from build123d import *

# Parameters (mm, degrees)
SKETCH_2_R          = 6.5
EXTRUDE_1_DEPTH     = 2.5
SKETCH_3_R          = 2.1
CUT_EXTRUDE_1_DEPTH = 2.5
CUT_EXTRUDE_2_DEPTH = 10
SKETCH_5_R          = 2.2
CUT_EXTRUDE_3_DEPTH = 10
CUT_EXTRUDE_4_DEPTH = 10


with BuildPart() as part:
    # 草图2 → 凸台-拉伸1 (new body)
    with BuildSketch(Plane(origin=(0, 0, 0), x_dir=(1, 0, 0), z_dir=(0, 1, 0))):
        with BuildLine():
            ThreePointArc((-47.091925455, 9.778744699), (-55, -1.253e-06), (-47.091923006, -9.778745223))
            ThreePointArc((-47.091923006, -9.778745223), (-33.750000065, -19.485571473), (-32.014603203, -35.893428778))
            ThreePointArc((-32.014603203, -35.893428778), (-27.500000081, -47.631397162), (-15.077319674, -45.672174193))
            ThreePointArc((-15.077319674, -45.672174193), (-9.8e-08, -38.97114317), (15.077319542, -45.672174048))
            ThreePointArc((15.077319542, -45.672174048), (27.500000118, -47.63139714), (32.014603117, -35.893428511))
            ThreePointArc((32.014603117, -35.893428511), (33.750000078, -19.485571451), (47.091922781, -9.778745271))
            ThreePointArc((47.091922781, -9.778745271), (55, -2.05e-07), (47.091923183, 9.778745185))
            ThreePointArc((47.091923183, 9.778745185), (33.750000105, 19.485571404), (32.01460321, 35.893428798))
            ThreePointArc((32.01460321, 35.893428798), (27.499999984, 47.631397217), (15.077319539, 45.672174044))
            ThreePointArc((15.077319539, 45.672174044), (1.8e-08, 38.97114317), (-15.077319515, 45.672174018))
            ThreePointArc((-15.077319515, 45.672174018), (-27.5000001, 47.63139715), (-32.014603117, 35.893428511))
            ThreePointArc((-32.014603117, 35.893428511), (-33.750000761, 19.485570266), (-47.091925455, 9.778744699))
        make_face()
        with Locations(Location((0, 0, 0), (0, 0, 270))):
            Circle(SKETCH_2_R, mode=Mode.SUBTRACT)
    extrude(amount=EXTRUDE_1_DEPTH)

    # 草图3 → 切除-拉伸1 (cut)
    with BuildSketch(Plane(origin=(0, 2.5, 0), x_dir=(1, 0, 0), z_dir=(0, 1, 0))):
        with Locations(Location((-22.5, 38.97114317, 0), (0, 0, 270))):
            Circle(SKETCH_3_R)
        with Locations(Location((22.5, 38.97114317, 0), (0, 0, 270))):
            Circle(SKETCH_3_R)
        with Locations(Location((45, 0, 0), (0, 0, 270))):
            Circle(SKETCH_3_R)
        with Locations(Location((22.5, -38.97114317, 0), (0, 0, 270))):
            Circle(SKETCH_3_R)
        with Locations(Location((-22.5, -38.97114317, 0), (0, 0, 270))):
            Circle(SKETCH_3_R)
        with Locations(Location((-45, 0, 0), (0, 0, 270))):
            Circle(SKETCH_3_R)
    extrude(amount=-CUT_EXTRUDE_1_DEPTH, mode=Mode.SUBTRACT)

    # 草图4 → 切除-拉伸2 (cut)
    with BuildSketch(Plane(origin=(0, 2.5, 0), x_dir=(1, 0, 0), z_dir=(0, 1, 0))):
        Polygon((-21.320889551, 23.855935356), (13.529450533, 3.223344728), (3.340516889, -13.986699758), (-31.509823195, 6.64589087), align=None)
    extrude(amount=-CUT_EXTRUDE_2_DEPTH, mode=Mode.SUBTRACT)

    # 草图5 → 切除-拉伸3 (cut)
    with BuildSketch(Plane(origin=(0, 2.5, 0), x_dir=(1, 0, 0), z_dir=(0, 1, 0))):
        with Locations(Location((14.424226019, -3.116953122, 0), (0, 0, 270))):
            Circle(SKETCH_5_R)
        with Locations(Location((9.329759197, -11.721975365, 0), (0, 0, 270))):
            Circle(SKETCH_5_R)
        with Locations(Location((-27.310131859, 21.591210963, 0), (0, 0, 270))):
            Circle(SKETCH_5_R)
        with Locations(Location((-32.404598681, 12.98618872, 0), (0, 0, 270))):
            Circle(SKETCH_5_R)
    extrude(amount=-CUT_EXTRUDE_3_DEPTH, mode=Mode.SUBTRACT)

    # 草图6 → 切除-拉伸4 (cut)
    with BuildSketch(Plane(origin=(0, 2.5, 0), x_dir=(1, 0, 0), z_dir=(0, 1, 0))):
        Polygon((-32.518067513, 17.701814323), (-31.499174149, 19.422818771), (14.537694851, -7.832578725), (13.518801487, -9.553583174), align=None)
    extrude(amount=-CUT_EXTRUDE_4_DEPTH, mode=Mode.SUBTRACT)


solid = part.part
CAD build for the part. Positions are in the model's coordinates, mm. A direction names the side the tool comes from. Round coordinates to 2 decimals unless told otherwise and drop trailing zeros. Write each loop counter-clockwise with the first axis right and the second up, starting at its lowest first coordinate (ties: lowest second). Pieces come first, ordered by that corner, then holes. Notation, with made-up numbers: (79, -40) -> (100, -40) arc R18 cw to (100, -19) -> close; hole circle Ø1 at (54.5, -22.75). An arc over 180 degrees is marked (long way). Answer as a JSON object with one key per item and string values.
(1) Two-plate mould, pull along Z, no slides. Class faces 1 (the face through (-20.418, 1.268, -39.245)), 2 (the face through (0.238, 1.232, -38.973)), 3 (the face through (55, 1, 0)): +Z half, -Z half, draft (parallel to the pull), parting line (faces both ways), or undercut.
Reported:
{"face 1": "undercut", "face 2": "-Z half", "face 3": "parting line"}
(2) Band-saw the part on C-C, the plane y = 0.4. Count the separate pieces of the cut face and the enclosed holes in it, then the cut area to 3 significant figures.
Reported:
{"separate pieces": "1", "enclosed holes": "11", "area": "5,770 mm^2"}
(3) Probe probe 1 along X at (y, z) = (0.6, -11.5); probe 2 along X at (y, z) = (2.1, -16.5); probe 3 along Z at (x, y) = (11, 2.3). List the from-to ranges inside material, lowest first. Write a range as [from, to].
Reported:
{"probe 1": "x = [-42.2, -34.03], [-30.78, -28.64], [-0.45, 42.2]", "probe 2": "x = [-35.85, -30.49], [-26.56, -25.68], [-8.9, 35.85]", "probe 3": "z = [-42.21, -4.72], [1.05, 5.74], [8.06, 10.29], [13.15, 42.21]"}
(4) Band-saw the part on B-B, the plane x = 45. List the corners of the cut face in (y, z), then the cut area to 3 significant figures.
Reported:
{"outline": "(0, -10.34) -> (2.5, -10.34) -> (2.5, -2.1) -> (0, -2.1) -> close; (0, 2.1) -> (2.5, 2.1) -> (2.5, 10.34) -> (0, 10.34) -> close", "area": "41.2 mm^2"}
(5) Band-saw the part on D-D, the plane x = -22.5. List the corners of the cut face in (y, z), then the cut area to 3 significant figures.
Reported:
{"outline": "(0, -48.97) -> (2.5, -48.97) -> (2.5, -41.07) -> (0, -41.07) -> close; (0, -36.87) -> (2.5, -36.87) -> (2.5, -21.86) -> (0, -21.86) -> close; (0, -1.31) -> (2.5, -1.31) -> (2.5, 36.87) -> (0, 36.87) -> close; (0, 41.07) -> (2.5, 41.07) -> (2.5, 48.97) -> (0, 48.97) -> close", "area": "172 mm^2"}
(6) Which spindle directions (+Z, -Z, +X, -X, +Y, -Y) get a long thin tool onto all of the face, cutting with end or side? Do faces 4 (the face through (-29.68, 1.27, -16.02)), 5 (the face through (11, 2.5, 10)). Say none if no direction does.
Reported:
{"face 4": "+Y, -Y", "face 5": "+Z, -Z, +X, -X, +Y"}
(7) Band-saw the part on A-A, the plane x = 22.5. List the corners of the cut face in (y, z), then the cut area to 3 significant figures.
Reported:
{"outline": "(0, -48.97) -> (2.5, -48.97) -> (2.5, -41.07) -> (0, -41.07) -> close; (0, -36.87) -> (2.5, -36.87) -> (2.5, 36.87) -> (0, 36.87) -> close; (0, 41.07) -> (2.5, 41.07) -> (2.5, 48.97) -> (0, 48.97) -> close", "area": "224 mm^2"}
(8) Pin check, flat tips, straight feed: P1, Ø6.5, axis at x = -45, z = 0, coming from the +Y side; P2, Ø1.5, axis at x = -42.5, y = 1.5, coming from the -Z side. Stop position of each tip, or through.
Reported:
{"P1": "stops at y = 2.5", "P2": "stops at z = -11.74"}
